from build123d import *

# Parameters (mm, degrees)
SKETCH_1_W            = 121.11
SKETCH_1_H            = 77.93
EXTRUDE_1_DEPTH       = 1.5
HOLE_WIZARD_2_0_2_1_D = 2
SKETCH_4_W            = 120.11
SKETCH_4_H            = 76
EXTRUDE_2_DEPTH       = 5
SKETCH_5_W            = 118.11
SKETCH_5_H            = 70.5
EXTRUDE_3_DEPTH       = 1


with BuildPart() as part:
    # 草图1 → 凸台-拉伸1 (new body)
    with BuildSketch(Plane.XY):
        with Locations((60.555, 38.965)):
            Rectangle(SKETCH_1_W, SKETCH_1_H)
    extrude(amount=EXTRUDE_1_DEPTH)

    # Ø2.0 (2) 直径孔1 (through all)
    with Locations(Plane.XY.offset(1.5)):
        with Locations((23.02, 74.29), (23.02, 5), (116.11, 74.29), (116.11, 5)):
            Hole(HOLE_WIZARD_2_0_2_1_D / 2)

    # 草图4 → 凸台-拉伸2 (add)
    with BuildSketch(Plane.XY.offset(1.5)):
        with Locations((60.555, 39)):
            Rectangle(SKETCH_4_W, SKETCH_4_H)
    extrude(amount=EXTRUDE_2_DEPTH)

    # 草图5 → 凸台-拉伸3 (add)
    with BuildSketch(Plane.XY.offset(6.5)):
        with Locations((60.555, 40.75)):
            Rectangle(SKETCH_5_W, SKETCH_5_H)
    extrude(amount=EXTRUDE_3_DEPTH)


solid = part.part
Check sheet for the modelled part. Datum: model origin and axes. Units: mm. A direction names the side the tool comes from. Coordinates: 2 decimals unless noted, no trailing zeros. Write each loop counter-clockwise with the first axis right and the second up, starting at its lowest first coordinate (ties: lowest second). Pieces come first, ordered by that corner, then holes.
Item 1: Cross-section at B-B on z = 4.5. Record the boundary of the cut face in (x, y).
Numbers:
outline: (0.5, 1) - (120.61, 1) - (120.61, 77) - (0.5, 77) - close
Item 2: Access from +Z, -Z, +X, -X, +Y, -Y to the whole of each face (thin tool, end or side, straight path). Record for faces 1 (the face through (120.61, 38, 4)), 2 (the face through (60, 1, 4)), 3 (the face through (0.5, 38, 4)).
Numbers:
face 1: +Z, +X, +Y, -Y
face 2: +Z, +X, -X, -Y
face 3: +Z, -X, +Y, -Y
Item 3: Cross-section at A-A on x = 29.5. Record the boundary of the cut face in (y, z).
Numbers:
outline: (0, 0) - (77.93, 0) - (77.93, 1.5) - (77, 1.5) - (77, 6.5) - (76, 6.5) - (76, 7.5) - (5.5, 7.5) - (5.5, 6.5) - (1, 6.5) - (1, 1.5) - (0, 1.5) - close
Item 4: Scan lines: probe 1 along Y at (x, z) = (23.02, 0.5); probe 2 along X at (y, z) = (74.29, 0.9); probe 3 along X at (y, z) = (38, 6.75). Record each from-to range of solid material in increasing order.
Numbers:
probe 1: y = 0 to 4, 6 to 73.29, 75.29 to 77.93
probe 2: x = 0 to 22.02, 24.02 to 115.11, 117.11 to 121.11
probe 3: x = 1.5 to 119.61
Item 5: Depth check by flat-ended pin: pin 1 Ø1.5 at (x, z) = (82.5, 4.5) entering from +Y; pin 2 Ø0.8 at (y, z) = (57.5, 7) entering from -X; pin 3 Ø1 at (x, y) = (23, 5) entering from -Z. Enter the tip coordinate at first touch or a pass-through.
Numbers:
pin 1: stops at y = 77
pin 2: stops at x = 1.5
pin 3: stops at z = 1.5
